Can you work these out from the model? Positions are in its coordinate system, mm. A direction names the side the tool comes from. Coordinates: 2 decimals unless noted, no trailing zeros. Order: outer loops, then holes, each group sorted by start corner. A loop starts at its lowest first (then second) coordinate and runs counter-clockwise, first axis right, second up. Notation, with made-up numbers: (27, 57) -> (75, 57) arc R20 cw to (75, 91) -> close; hole circle Ø8 at (2, 22.5). An arc over 180 degrees is marked (long way). Answer in a Markdown table with one row per item. Add a question column.
1. Imagine slicing it at D-D on y = -34.5. Write out the boundary of the cut face in (x, z).
2. Will these pins go through, and if not, where does the flat tip stop? pin 1 (6 mm diameter, centred on x = 8.5, z = 36.5, fed in from -Y); pin 2 (8 mm diameter, centred on y = 11, z = 71.5, fed in from -X); pin 3 (12 mm diameter, centred on x = 12, y = 3, fed in from -Z); pin 4 (12 mm diameter, centred on y = 21.5, z = 26, fed in from +X).
3. Imagine slicing it at B-B on y = 14. Write out the boundary of the cut face in (x, z), plus the area to 3 significant figures.
4. Imagine slicing it at C-C on x = 15.5. Write out the boundary of the cut face in (y, z).
5. Imagine slicing it at A-A on z = 61.5. Write out the boundary of the cut face in (x, y).
6. On a 3-axis mill with a long thin cutter (end or side, diameter ignored), from which of +Z, -Z, +X, -X, +Y, -Y can I reach the whole of each face in a straight line? I mean faces 1 (the face through (5, -42.026, 52)), 2 (the face through (-8.577, -11, 44)), 3 (the face through (4.928, -10.986, 63.544)). Say none if no direction works.
7. We'd pull the mould along X, two halves only. Please class faces 4 (the face through (33.867, -3, 9)), 5 (the face through (5, 11.898, 57)), 6 (the face through (5.476, 56.436, 9.392)): pulls with the +X half, pulls with the -X half, needs draft (parallel to the pull), parting line crosses it, or undercut.
8. If I drill on line 1 along Y through (x, z) = (-2, 59); line 2 along Y through (x, z) = (-2, 77); line 3 along Z through (x, y) = (24, 70.5), over which ranges is the centre line in solid material (lowest first)? Write a range as [from, to].
from build123d import *

# Parameters (mm, degrees)
F0_R      = 11.2267046734
F0_R_2    = 11.0852071495
F1_DEPTH  = 19.05
F2_W      = 26.7343660817
F2_H      = 81.4062468708
F3_DEPTH  = 50.8
F5_DEPTH  = 42.4459602142
F6_R      = 6.3073673096
F7_DEPTH  = 27.432
F8_DEPTH  = 136.6678641567
F9_R      = 5.937984747
F10_DEPTH = 30.734


with BuildPart() as f1:
    # F0 (on Top) → F1 (new body)
    with BuildSketch(Plane.XY):
        with BuildLine():
            Line((-18.1084536016, 67.2573745251), (-18.1084536016, -71.298904717))
            ThreePointArc((-18.1084536016, -71.298904717), (7.8795179725, -97.286876291), (33.8674895465, -71.298904717))
            Line((33.8674895465, -71.298904717), (33.8674895465, 67.2573745251))
            ThreePointArc((33.8674895465, 67.2573745251), (7.8795179725, 93.2453460991), (-18.1084536016, 67.2573745251))
        make_face()
        with Locations((7.8795179725, -71.298904717)):
            Circle(F0_R, mode=Mode.SUBTRACT)
        with Locations((7.8795179725, 67.2573745251)):
            Circle(F0_R_2, mode=Mode.SUBTRACT)
    extrude(amount=F1_DEPTH)

    # F2 (on face) → F3 (join)
    with BuildSketch(Plane.XY.offset(19.05)):
        with Locations((4.7897123732, -1.3231355697)):
            Rectangle(F2_W, F2_H)
    extrude(amount=F3_DEPTH)

    # F4 (on face) → F5 (cut, through all)
    with BuildSketch(Plane(origin=(-8.5774706677, 0, 0), x_dir=(0, -1, 0), z_dir=(-1, 0, 0))):
        with BuildLine():
            Line((10.6878159568, 69.85), (-11.8984412402, 69.85))
            Line((-11.8984412402, 69.85), (-11.8984412402, 42.8989976645))
            ThreePointArc((-11.8984412402, 42.8989976645), (-0.6053126417, 31.605869066), (10.6878159568, 42.8989976645))
            Line((10.6878159568, 42.8989976645), (10.6878159568, 69.85))
        make_face()
    extrude(amount=-F5_DEPTH, mode=Mode.SUBTRACT)

    # F6 (on face) → F7 (join)
    with BuildSketch(Plane(origin=(0, 39.3799878657, 0), x_dir=(-1, 0, 0), z_dir=(0, 1, 0))):
        with Locations((-4.7897123732, 69.85)):
            Circle(F6_R)
        with BuildLine():
            Line((1.5176549365, 69.85), (8.5774706677, 69.85))
            ThreePointArc((8.5774706677, 69.85), (-4.7897123732, 83.2171830408), (-18.156895414, 69.85))
            Line((-18.156895414, 69.85), (-11.0970796828, 69.85))
            ThreePointArc((-11.0970796828, 69.85), (-4.7897123732, 76.1573673096), (1.5176549365, 69.85))
        make_face()
    extrude(amount=-F7_DEPTH)

    # F6 (on face) → F8 (cut, through all)
    with BuildSketch(Plane(origin=(0, 39.3799878657, 0), x_dir=(-1, 0, 0), z_dir=(0, 1, 0))):
        with BuildLine():
            ThreePointArc((-11.0970796828, 69.85), (-4.7897123732, 63.5426326904), (1.5176549365, 69.85))
            Line((1.5176549365, 69.85), (-11.0970796828, 69.85))
        make_face()
        with BuildLine():
            Line((-11.0970796828, 69.85), (1.5176549365, 69.85))
            ThreePointArc((1.5176549365, 69.85), (-4.7897123732, 76.1573673096), (-11.0970796828, 69.85))
        make_face()
    extrude(amount=-F8_DEPTH, mode=Mode.SUBTRACT)

    # F9 (on face) → F10 (join)
    with BuildSketch(Plane.XZ.offset(42.0262590051)):
        with BuildLine():
            Line((11.0970796828, 69.85), (18.156895414, 69.85))
            ThreePointArc((18.156895414, 69.85), (4.7897123732, 83.2171830408), (-8.5774706677, 69.85))
            Line((-8.5774706677, 69.85), (-1.5176549365, 69.85))
            ThreePointArc((-1.5176549365, 69.85), (4.7897123732, 63.5426326904), (11.0970796828, 69.85))
        make_face()
        with Locations((4.7897123732, 69.85)):
            Circle(F9_R, mode=Mode.SUBTRACT)
    extrude(amount=-F10_DEPTH)


solid = f1.part
Answers follow:
| question | item | result |
|---|---|---|
| 1 | outline | (-18.11, 0) -> (33.87, 0) -> (33.87, 19.05) -> (18.16, 19.05) -> (18.16, 69.85) arc R13.37 ccw to (-8.58, 69.85) -> (-8.58, 19.05) -> (-18.11, 19.05) -> close; hole circle Ø11.88 at (4.79, 69.85) |
| 2 | pin 1 | stops at y = -42.03 |
| 2 | pin 2 | stops at x = -8.58 |
| 2 | pin 3 | stops at z = 0 |
| 2 | pin 4 | stops at x = 18.16 |
| 3 | outline | (-18.11, 0) -> (33.87, 0) -> (33.87, 19.05) -> (18.16, 19.05) -> (18.16, 69.85) arc R13.37 ccw to (-8.58, 69.85) -> (-8.58, 19.05) -> (-18.11, 19.05) -> close; hole circle Ø12.61 at (4.79, 69.85) |
| 3 | area | 2,500 mm² |
| 4 | outline | (-96.14, 0) -> (-79.54, 0) -> (-79.54, 19.05) -> (-96.14, 19.05) -> close; (-63.05, 0) -> (59.21, 0) -> (59.21, 19.05) -> (39.38, 19.05) -> (39.38, 77.85) -> (11.95, 77.85) -> (11.95, 69.85) -> (11.9, 69.85) -> (11.9, 42.9) arc R11.29 cw to (-10.69, 42.9) -> (-10.69, 69.85) -> (-11.29, 69.85) -> (-11.29, 77.85) -> (-42.03, 77.85) -> (-42.03, 19.05) -> (-63.05, 19.05) -> close; (75.31, 0) -> (92.1, 0) -> (92.1, 19.05) -> (75.31, 19.05) -> close |
| 5 | outline | (-8.58, -42.03) -> (18.16, -42.03) -> (18.16, -10.69) -> (-8.58, -10.69) -> close; (-8.58, 11.9) -> (18.16, 11.9) -> (18.16, 39.38) -> (-8.58, 39.38) -> close |
| 6 | face 1 | +Z, +X, -X, -Y |
| 6 | face 2 | +Z, -X, +Y, -Y |
| 6 | face 3 | +Z, +Y |
| 7 | face 4 | pulls with the +X half |
| 7 | face 5 | needs draft |
| 7 | face 6 | undercut |
| 8 | line 1 | y = [-42.03, -10.69], [11.9, 39.38] |
| 8 | line 2 | y = [-42.03, -11.29], [11.95, 39.38] |
| 8 | line 3 | z = [0, 19.05] |
